Study the drawing (mm; zero at the part's minimum x, y, z) and answer. Round coordinates to 2 decimals unless told otherwise and drop trailing zeros. Loops run counter-clockwise (first coordinate to the right, second up) from the corner with the lowest first, then second, coordinate; pieces in that order, holes last. Notation, with made-up numbers: M 60.25,59.5 L 107.25,59.5 A11 ccw 107.25,64.5 Z; hole C -36,67.5 d3. An arc over 180 degrees is marked long. Put each result on its own line as item: value. Start each with the question number.
(1) Section D-D, the plane y = 5.5 is taken. Determine the outline of the cut face in (x, z).
(2) Straight lines are drawn through the part: line 1 (Y direction, x = 38.5, z = 0.7); line 2 (X direction, y = 27, z = 0.3); line 3 (Y direction, x = 74, z = 0.1). For each, find the intervals that lie inside material, in ascending order.
(3) Section B-B, the plane x = 43 is taken. Determine the outline of the cut face in (y, z).
(4) Section C-C, the plane x = 84.5 is taken. Determine the outline of the cut face in (y, z).
(5) Section A-A, the plane y = 20 is taken. Determine the outline of the cut face in (x, z), then the cut area to 3 significant figures.
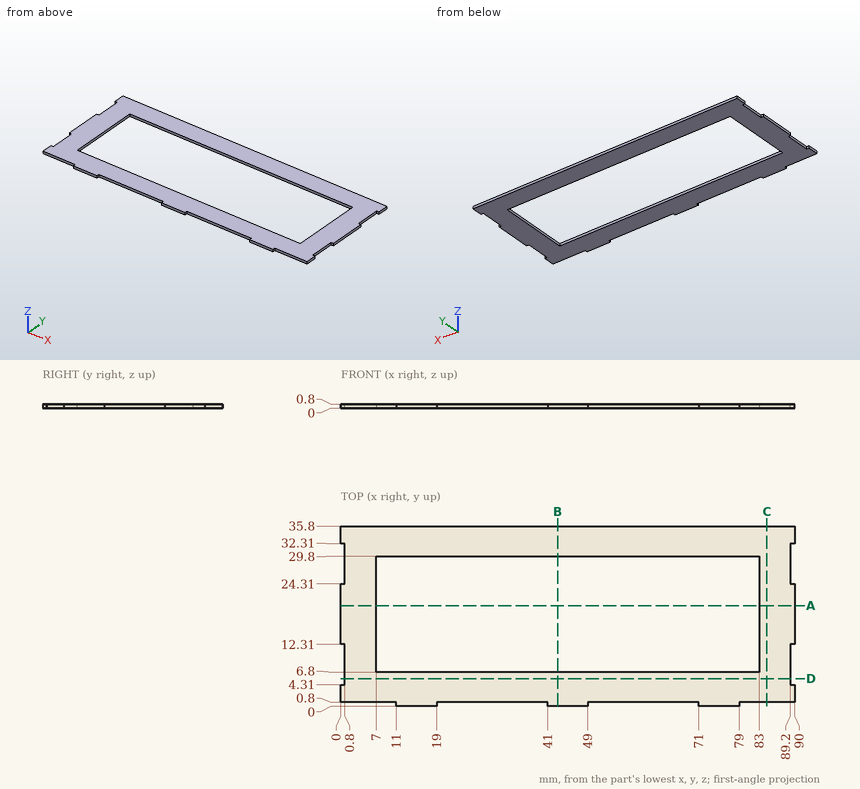
Recorded:
1. outline: M 0.8,0 L 89.2,0 L 89.2,0.8 L 0.8,0.8 Z
2. line 1: y = 0.8 to 6.8, 29.8 to 35.8
2. line 2: x = 0.8 to 7, 83 to 89.2
2. line 3: y = 0 to 6.8, 29.8 to 35.8
3. outline: M 0,0 L 6.8,0 L 6.8,0.8 L 0,0.8 Z; M 29.8,0 L 35.8,0 L 35.8,0.8 L 29.8,0.8 Z
4. outline: M 0.8,0 L 35.8,0 L 35.8,0.8 L 0.8,0.8 Z
5. outline: M 0,0 L 7,0 L 7,0.8 L 0,0.8 Z; M 83,0 L 90,0 L 90,0.8 L 83,0.8 Z
5. area: 11.2 mm²
